Build history of the part. All positions in model axes, mm. A direction names the side the tool comes from. Round coordinates to 2 decimals unless told otherwise and drop trailing zeros. Order: outer loops, then holes, each group sorted by start corner. A loop starts at its lowest first (then second) coordinate and runs counter-clockwise, first axis right, second up. Notation, with made-up numbers: (1.5, 49.25) - (10.5, 49.25) arc R19 cw to (10.5, 73.25) - close; hole circle Ø10 at (-38, 86.25). An arc over 180 degrees is marked (long way). One line per question, with ' | ' between items. Start each with the question number.
from build123d import *

# Parameters (mm, degrees)
SKETCH1_W           = 4.572
SKETCH1_H           = 28.575
SKETCH2_R           = 12.1666
BOSS_EXTRUDE1_DEPTH = 20.828
CUT_EXTRUDE1_DEPTH  = 26.4
HOLE1_D             = 5.1816
HOLE1_DEPTH         = 4.572
CIRPATTERN1_COUNT   = 6


with BuildPart() as part:
    # Sketch1 → Revolve1 (revolve)
    with BuildSketch(Plane(origin=(0, 0, 0), x_dir=(-1, 0, 0), z_dir=(0, 0, -1))):
        with Locations((15.321066246, 14.2875)):
            Rectangle(SKETCH1_W, SKETCH1_H)
    revolve(axis=Axis((-13.035066246, 0, 0), (-1, 0, 0)))

    # Sketch2 → Boss-Extrude1 (add)
    with BuildSketch(Plane(origin=(-13.035066246, 0, 0), x_dir=(0, 0, -1), z_dir=(1, 0, 0))):
        Circle(SKETCH2_R)
    extrude(amount=BOSS_EXTRUDE1_DEPTH)

    # Sketch3 → Cut-Extrude1 (cut, through all)
    with BuildSketch(Plane(origin=(7.792933754, 0, 0), x_dir=(0, 0, -1), z_dir=(1, 0, 0))):
        Polygon((0, -7.361697812), (6.3754, -3.680858906), (6.3754, 3.680818906), (0, 7.361657812), (-6.3754, 3.680818906), (-6.3754, -3.680858906), align=None)
    extrude(amount=-CUT_EXTRUDE1_DEPTH, mode=Mode.SUBTRACT)

    # Hole1
    with Locations(Plane(origin=(-13.035066246, 0, 0), x_dir=(0, 0, -1), z_dir=(1, 0, 0))):
        with Locations((-23.8125, 0)):
            hole1 = Hole(HOLE1_D / 2, depth=HOLE1_DEPTH)

    # CirPattern1: Hole1 ×6 about axis
    cirpattern1_axis = Axis((0, 0, 0), (1, 0, 0))
    for i in range(1, CIRPATTERN1_COUNT):
        add(hole1.rotate(cirpattern1_axis, i * 360 / CIRPATTERN1_COUNT), mode=Mode.SUBTRACT)


solid = part.part
Item 1: Slice it at C-C (y = -6.5). Write the cut outline in (x, z), plus the area to 3 significant figures.
Item 2: Slice it at B-B (x = -1). Write the cut outline in (y, z).
Item 3: Slice it at A-A (y = 0). Write the cut outline in (x, z) (3 decimals).
Item 4: Pin check, flat tips, straight feed: pin 1 (1 mm diameter, centred on x = -7.5, z = 7.5, fed in from -Y); pin 2 (10 mm diameter, centred on x = 3, y = -11.5, fed in from +Z); pin 3 (8 mm diameter, centred on y = 13.5, z = -20, fed in from +X). Stop position of each tip, or through.
Item 5: Wall check: line 1 along X through (y, z) = (8.5, 23); line 2 along Z through (x, y) = (-14, 20.5); line 3 along Z through (x, y) = (-13.5, -7). Give the ranges that are in metal, low to high. Write a range as [from, to].
Item 6: Pull direction Z, two halves, no side cores. Call faces 1 (the face through (-5, 0, -6.375)), 2 (the face through (-3, 12, 2)), 3 (the face through (-17.607, 0, -7)): released by +Z, released by -Z, zero draft, split by the parting line, or undercut.
Item 7: 3-axis set-ups, long thin cutter, end or side, ignore diameter. For faces 4 (the face through (-13.035, -12, 6)), 5 (the face through (7.793, -5, -5)), 6 (the face through (-4.73, 5.55, 3.14)): which of +Z, -Z, +X, -X, +Y, -Y reach the whole face in a straight line?
Item 8: Slice it at D-D (z = 2.5). Write the cut outline in (x, y), plus the area to 3 significant figures.
A:
1) outline: (-17.61, -27.83) - (-13.04, -27.83) - (-13.04, -10.28) - (7.79, -10.28) - (7.79, -1.49) - (-17.61, -1.49) - close; (-17.61, 1.49) - (7.79, 1.49) - (7.79, 10.28) - (-13.04, 10.28) - (-13.04, 27.83) - (-17.61, 27.83) - close | area: 607 mm^2
2) outline: circle Ø24.33 at (0, 0); hole (-7.36, 0) - (-3.68, -6.38) - (3.68, -6.38) - (7.36, 0) - (3.68, 6.38) - (-3.68, 6.38) - close
3) outline: (-17.607, -28.575) - (-13.035, -28.575) - (-13.035, -26.403) - (-17.607, -26.403) - close; (-17.607, -21.222) - (-13.035, -21.222) - (-13.035, -12.167) - (7.793, -12.167) - (7.793, -6.375) - (-17.607, -6.375) - close; (-17.607, 6.375) - (7.793, 6.375) - (7.793, 12.167) - (-13.035, 12.167) - (-13.035, 21.222) - (-17.607, 21.222) - close; (-17.607, 26.403) - (-13.035, 26.403) - (-13.035, 28.575) - (-17.607, 28.575) - close
4) pin 1: y = -9.95 | pin 2: z = 10.28 | pin 3: x = -13.04
5) line 1: [-17.61, -13.04] | line 2: [-19.91, -14.49], [-9.32, 9.32], [14.49, 19.91] | line 3: [-27.7, -0.63], [0.63, 27.7]
6) face 1: undercut | face 2: split by the parting line | face 3: zero draft
7) face 4: +X | face 5: +Z, -Z, +X, +Y, -Y | face 6: +X, -X
8) outline: (-17.61, -28.47) - (-13.04, -28.47) - (-13.04, -11.91) - (7.79, -11.91) - (7.79, -5.92) - (-17.61, -5.92) - close; (-17.61, 5.92) - (7.79, 5.92) - (7.79, 11.91) - (-13.04, 11.91) - (-13.04, 28.47) - (-17.61, 28.47) - close | area: 456 mm^2
